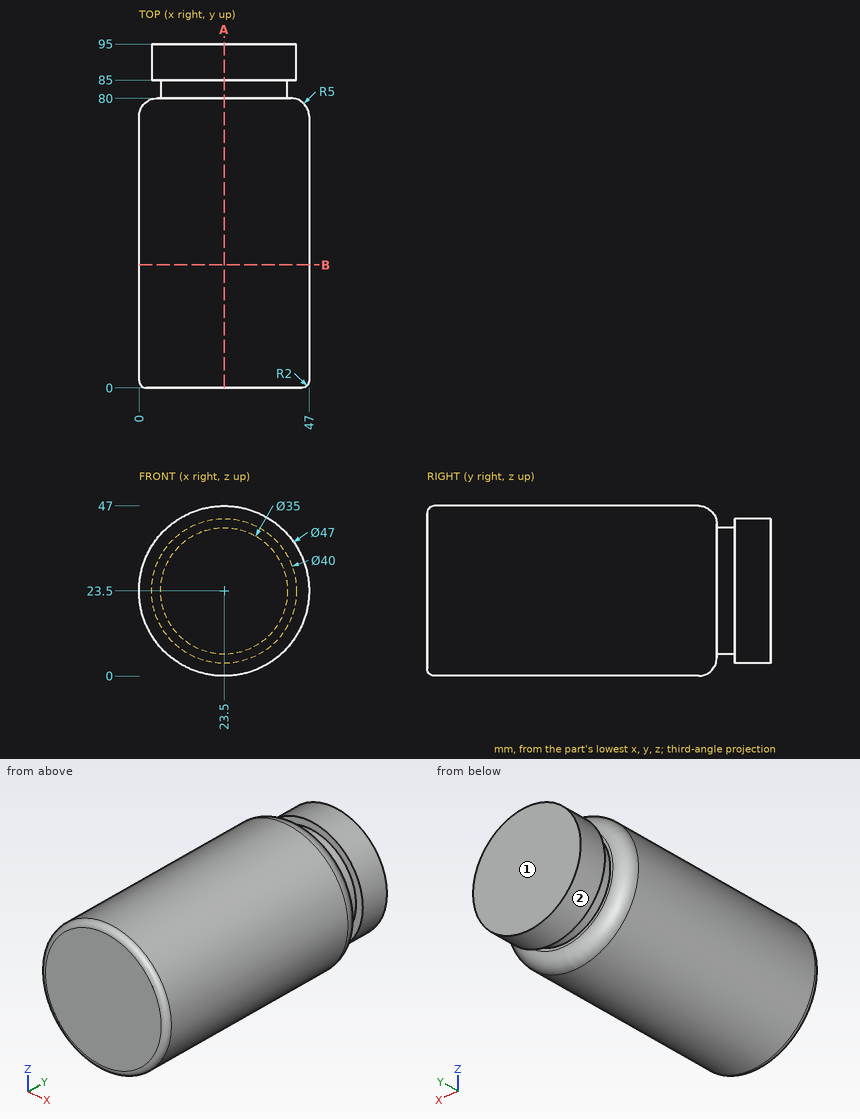
Verification items for this drawing (mm, ordinates from the low corner). A direction names the side the tool comes from. Coordinates: 2 decimals unless noted, no trailing zeros. Loops run counter-clockwise (first coordinate to the right, second up) from the corner with the lowest first, then second, coordinate; pieces in that order, holes last. Notation, with made-up numbers: (56.25, -22.75) - (107.25, -22.75) arc R22 cw to (107.25, 14.25) - close; hole circle Ø10 at (23.25, 14). An arc over 180 degrees is marked (long way). Use one line per item in the form item = value. Start each with the question number.
Item 1: Section check A-A, the plane x = 23.5. Enter the section's corners in (y, z), and give its area (3 significant figures).
Item 2: Section check B-B, the plane y = 34. Enter the section's corners in (x, z), and give its area (3 significant figures).
Item 3: Tool access check on the marked faces 1 and 2. Record the directions out of +Z, -Z, +X, -X, +Y, -Y that give a thin tool (end or side, any length) a straight path to the whole face; none if there is none.
Item 4: Thickness scan on probe 1 along Y at (x, z) = (17, 40); probe 2 along X at (y, z) = (10, 24); probe 3 along X at (y, z) = (5, 9). Record the ranges inside material, lowest first.
Item 5: Gauge pin test, flat ends, axial feed: pin 1 (8 mm diameter, centred on x = 4.5, z = 14.5, fed in from +Y); pin 2 (1.5 mm diameter, centred on y = 17.5, z = 38.5, fed in from -X); pin 3 (4 mm diameter, centred on y = 70.5, z = 34, fed in from -X); pin 4 (3 mm diameter, centred on y = 61, z = 10.5, fed in from -X). Record the tip position at first contact, or that the pin passes through.
Computed:
q1.outline = (0, 2) arc R2 ccw to (2, 0) - (75, 0) arc R5 ccw to (80, 5) - (80, 6) - (85, 6) - (85, 3.5) - (95, 3.5) - (95, 43.5) - (85, 43.5) - (85, 41) - (80, 41) - (80, 42) arc R5 ccw to (75, 47) - (2, 47) arc R2 ccw to (0, 45) - close
q1.area = 4,320 mm2
q2.outline = circle Ø47 at (23.5, 23.5)
q2.area = 1,730 mm2
q3.face_1 = +Z, -Z, +X, -X, +Y
q3.face_2 = +Y
q4.probe_1 = 0 to 80, 85 to 95
q4.probe_2 = 0.01 to 46.99
q4.probe_3 = 5.01 to 41.99
q5.pin_1 = 95
q5.pin_2 = 4.81
q5.pin_3 = 1.59
q5.pin_4 = 3.01
